Geometry check sheet. Reference: the model listing, model coordinates, mm. Round coordinates to 2 decimals unless told otherwise and drop trailing zeros. Order: outer loops, then holes, each group sorted by start corner. A loop starts at its lowest first (then second) coordinate and runs counter-clockwise, first axis right, second up. Notation, with made-up numbers: (13, -9) -> (25, -9) arc R29 cw to (25, 18) -> close; hole circle Ø9 at (-5.5, -27). An arc over 180 degrees is marked (long way). Answer as a JSON object with one key per item and string values. Group by question number.
from build123d import *

# Parameters (mm, degrees)
RESSALTO_EXTRUS_O1_DEPTH   = 300
RESSALTO_EXTRUS_O1_TAPER   = -20
CORTE_EXTRUS_O1_DEPTH      = 185.19107038
CORTE_EXTRUS_O1_DEPTH_BACK = 185.19107038


with BuildPart() as part:
    # Esboço1 → Ressalto-extrusão1 (new body)
    with BuildSketch(Plane.XY):
        with BuildLine():
            Line((75, -250), (75, 250))
            ThreePointArc((75, 250), (0, 325), (-75, 250))
            Line((-75, 250), (-75, -250))
            ThreePointArc((-75, -250), (0, -325), (75, -250))
        make_face()
    extrude(amount=RESSALTO_EXTRUS_O1_DEPTH, taper=RESSALTO_EXTRUS_O1_TAPER)

    # Esboço4 → Corte-extrusão1 (cut, two sides)
    with BuildSketch(Plane(origin=(0, 0, 0), x_dir=(0, 0, -1), z_dir=(1, 0, 0))) as corte_extrus_o1_sk:
        with BuildLine():
            Line((-329.933259094, 603.571428571), (-300, 803.571428571))
            Line((-300, 803.571428571), (-270.066740906, 603.571428571))
            add(Edge.make_bspline(
                [(-329.933259094, 603.571428571), (-391.958337138, 189.14894388), (-345.979168569, -447.42728801), (-300, -1084.0035199), (-254.020831431, -447.42728801), (-208.041662862, 189.14894388), (-270.066740906, 603.571428571)],
                knots=[3.663907475, 3.663907475, 3.663907475, 5.410092697, 5.410092697, 7.156277918, 7.156277918, 8.902463139, 8.902463139, 8.902463139], degree=2, weights=[1, 0.642459696, 1, 0.642459696, 1, 0.642459696, 1]))
        make_face()
    extrude(amount=CORTE_EXTRUS_O1_DEPTH, mode=Mode.SUBTRACT)
    extrude(corte_extrus_o1_sk.sketch, amount=-CORTE_EXTRUS_O1_DEPTH_BACK, mode=Mode.SUBTRACT)


solid = part.part
Item 1: Depth check by flat-ended pin: pin 1 Ø1 at (y, z) = (211.5, 127) entering from -X; pin 2 Ø8 at (y, z) = (124.5, 79.5) entering from -X; pin 3 Ø6 at (x, z) = (-29.5, 93) entering from +Y. Enter the tip coordinate at first touch or a pass-through.
Item 2: Sectioned sample at B-B, the plane z = 154.5. Enter the section's corners in (x, y).
Item 3: Thickness scan on L1, parallel to Z at x = 57.5, y = -1; L2, parallel to X at y = -217.5, z = 87; L3, parallel to X at y = 162.5, z = 22. Record the ranges inside material, lowest first.
Item 4: Sectioned sample at A-A, the plane z = 119. Enter the section's corners in (x, y), then the cut area to 3 significant figures.
Result:
{
 "1": {"pin 1": "stops at x = -121.41", "pin 2": "stops at x = -105.39", "pin 3": "stops at y = 356.17"},
 "2": {"outline": "(-131.23, -250) arc R131.23 ccw to (131.23, -250) -> (131.23, 250) arc R131.23 ccw to (-131.23, 250) -> close"},
 "3": {"L1": "z = 0 to 240", "L2": "x = -106.67 to 106.67", "L3": "x = -83.01 to 83.01"},
 "4": {"outline": "(-118.31, -250) arc R118.31 ccw to (118.31, -250) -> (118.31, 250) arc R118.31 ccw to (-118.31, 250) -> close", "area": "162,000 mm2"}
}
